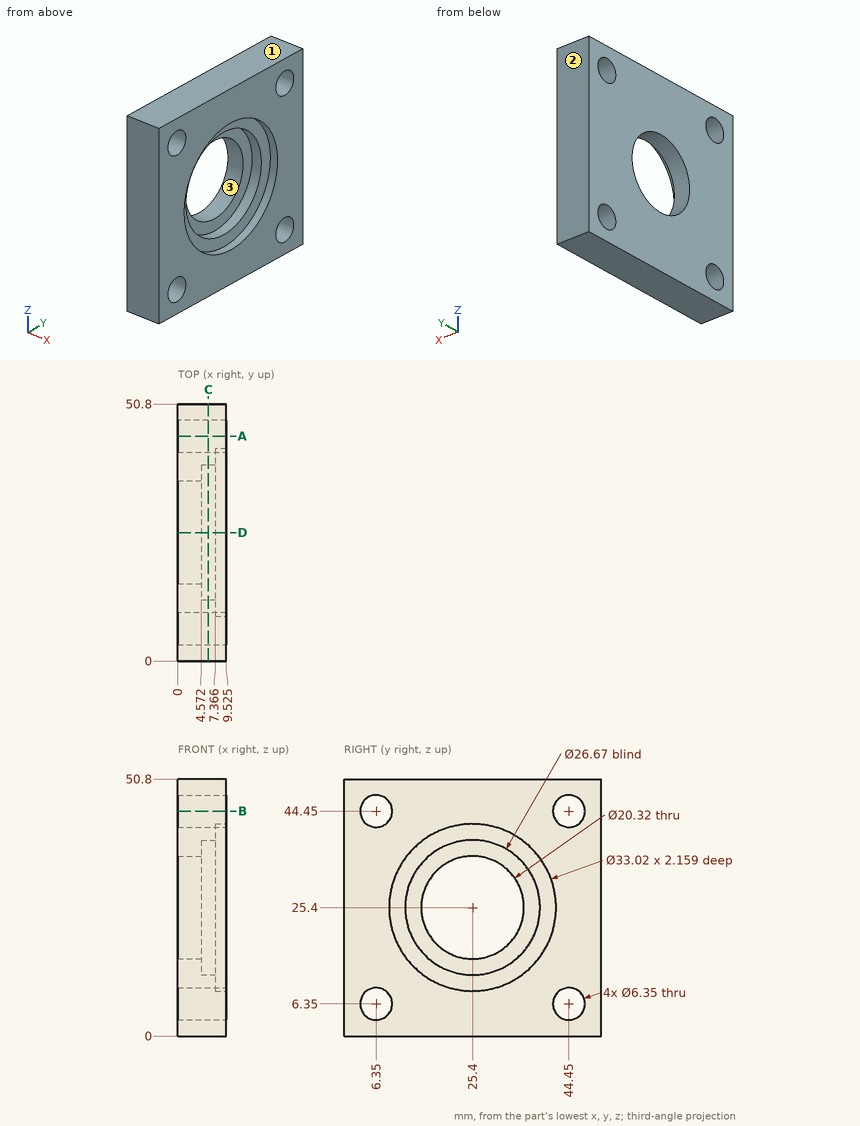
Study the drawing (mm; zero at the part's minimum x, y, z) and answer. Coordinates: 2 decimals unless noted, no trailing zeros. Write each loop counter-clockwise with the first axis right and the second up, starting at its lowest first coordinate (ties: lowest second). Pieces come first, ordered by that corner, then holes. Notation, with made-up numbers: M -28,62.25 L 29,62.25 A28 cw 29,95.25 Z; hole C 12,-10.75 d4. An arc over 180 degrees is marked long. Use a Markdown table: item, result. Add a question column.
1. For a pull along Z with two mould halves and no side action, classify the marked faces 1, 2 and 3 as +Z half, -Z half, draft (parallel to the pull), parting line (faces both ways), or undercut.
2. Straight lines are drawn through the part: line 1 along Z through (x, y) = (3.75, 6.35) (3 decimals); line 2 along Y through (x, z) = (7.25, 46); line 3 along Y through (x, z) = (4, 5.5). For each, find the intervals that lie inside material, in ascending order. Write a range as [from, to].
3. Section A-A (y = 44.45) is taken. Give the vertices of the cut face in (x, z) (3 decimals), plus the area to 3 significant figures.
4. Section C-C (x = 6) is taken. Give the vertices of the cut face in (y, z) (3 decimals), plus the area to 3 significant figures.
5. Section D-D (y = 25.4) is taken. Give the vertices of the cut face in (x, z) (3 decimals), plus the area to 3 significant figures.
Data:
| question | item | result |
|---|---|---|
| 1 | face 1 | +Z half |
| 1 | face 2 | draft |
| 1 | face 3 | undercut |
| 2 | line 1 | z = [0, 3.175], [9.525, 41.275], [47.625, 50.8] |
| 2 | line 2 | y = [0, 3.58], [9.12, 41.68], [47.22, 50.8] |
| 2 | line 3 | y = [0, 3.29], [9.41, 41.39], [47.51, 50.8] |
| 3 | outline | M 0,0 L 9.525,0 L 9.525,3.175 L 0,3.175 Z; M 0,9.525 L 9.525,9.525 L 9.525,41.275 L 0,41.275 Z; M 0,47.625 L 9.525,47.625 L 9.525,50.8 L 0,50.8 Z |
| 3 | area | 363 mm2 |
| 4 | outline | M 0,0 L 50.8,0 L 50.8,50.8 L 0,50.8 Z; hole C 6.35,6.35 d6.35; hole C 6.35,44.45 d6.35; hole C 25.4,25.4 d26.67; hole C 44.45,6.35 d6.35; hole C 44.45,44.45 d6.35 |
| 4 | area | 1,900 mm2 |
| 5 | outline | M 0,0 L 9.525,0 L 9.525,8.89 L 7.366,8.89 L 7.366,12.065 L 4.572,12.065 L 4.572,15.24 L 0,15.24 Z; M 0,35.56 L 4.572,35.56 L 4.572,38.735 L 7.366,38.735 L 7.366,41.91 L 9.525,41.91 L 9.525,50.8 L 0,50.8 Z |
| 5 | area | 245 mm2 |
